```python
from build123d import *

# Parameters (mm, degrees)
SKETCH_1_R          = 4.75
EXTRUDE_1_DEPTH     = 7
CUT_EXTRUDE_1_DEPTH = 4
SKETCH_3_R          = 1.85
CUT_EXTRUDE_2_DEPTH = 8
CUT_EXTRUDE_7_DEPTH = 2.5


with BuildPart() as part:
    # Эскиз1 → Бобышка-Вытянуть1 (new body)
    with BuildSketch(Plane(origin=(0, 0, 0), x_dir=(1, 0, 0), z_dir=(0, 1, 0))):
        Circle(SKETCH_1_R)
    extrude(amount=EXTRUDE_1_DEPTH)

    # Эскиз2 → Вырез-Вытянуть1 (cut)
    with BuildSketch(Plane(origin=(0, 7, 0), x_dir=(1, 0, 0), z_dir=(0, 1, 0))):
        Polygon((-3.181980515, 0), (-2.25, -0.931980515), (-2.25, -2.25), (-0.931980515, -2.25), (0, -3.181980515), (0.931980515, -2.25), (2.25, -2.25), (2.25, -0.931980515), (3.181980515, 0), (2.25, 0.931980515), (2.25, 2.25), (0.931980515, 2.25), (0, 3.181980515), (-0.931980515, 2.25), (-2.25, 2.25), (-2.25, 0.931980515), align=None)
    extrude(amount=-CUT_EXTRUDE_1_DEPTH, mode=Mode.SUBTRACT)

    # Эскиз3 → Вырез-Вытянуть2 (cut, through all)
    with BuildSketch(Plane.XZ):
        Circle(SKETCH_3_R)
    extrude(amount=-CUT_EXTRUDE_2_DEPTH, mode=Mode.SUBTRACT)

    # Эскиз4<3> → Вырез-Вытянуть7 (cut)
    with BuildSketch(Plane.XZ):
        with BuildLine():
            ThreePointArc((2.254348542, 4.180958341), (-1.817746304, 4.388427779), (-4.550449136, 1.362318854))
            Line((-4.550449136, 1.362318854), (2.254348542, 4.180958341))
        make_face()
        with BuildLine():
            Line((4.550449136, -1.362318854), (-2.254348542, -4.180958341))
            ThreePointArc((-2.254348542, -4.180958341), (1.817746304, -4.388427779), (4.550449136, -1.362318854))
        make_face()
    extrude(amount=-CUT_EXTRUDE_7_DEPTH, mode=Mode.SUBTRACT)


solid = part.part
```
Verification items for the finished model (mm, model axes). A direction names the side the tool comes from. Round coordinates to 2 decimals unless told otherwise and drop trailing zeros. Order: outer loops, then holes, each group sorted by start corner. A loop starts at its lowest first (then second) coordinate and runs counter-clockwise, first axis right, second up. Notation, with made-up numbers: (21, 67.25) - (25, 67.25) arc R20 ccw to (25, 90.25) - close; hole circle Ø5 at (54.5, 23.25). An arc over 180 degrees is marked (long way). Use CSV: the item, a comma, the result in double quotes. Start each with the question number.
1) Section check C-C, the plane z = 1.5. Record the cut outline in (x, y), plus the area to 3 significant figures.
2) Section check D-D, the plane x = 2.5. Record the cut outline in (y, z), plus the area to 3 significant figures.
3) Section check B-B, the plane x = 1.5. Record the cut outline in (y, z), plus the area to 3 significant figures.
4) Section check A-A, the plane y = 5.5. Record the cut outline in (x, z), plus the area to 3 significant figures.
5) Go/stop test with flat-tipped pins: P1, Ø3, axis at y = 5, z = 2, coming from the +X side; P2, Ø2, axis at y = 4, z = -2.5, coming from the +X side; P3, Ø1, axis at x = -2, z = 3.5, coming from the -Y side; P4, Ø4.5, axis at x = 0, z = 0, coming from the -Y side. Record where each tip stops, or that it passes through.
6) Mould release check, pull along Z, two halves, no side actions. Record for faces 6 (the flat face through (1.2, 1.23, -2.75)), 7 (the flat face through (-1.2, 1.23, 2.75)), 8 (the flat face through (-2.2, 0, -0.1)), 9 (the flat face through (2.25, 5, 2)): +Z half, -Z half, draft (parallel to the pull), parting line (faces both ways), or undercut.
7) Thickness scan on L1, parallel to Z at x = 0, y = 0.85; L2, parallel to Y at x = 2.5, z = -0.5; L3, parallel to X at y = 3.5, z = -0.5. Record the ranges inside material, lowest first.
8) Access from +Z, -Z, +X, -X, +Y, -Y to the whole of each face (thin tool, end or side, straight path). Record for faces 1 (the cylindrical face through (-4.745, 4.229, -0.209)), 2 (the flat face through (3, 7, 1)), 3 (the flat face through (-1, 2.5, 3)), 4 (the flat face through (2, 5, 2.25)), 5 (the flat face through (1, 2.5, -3)).
Answers:
1,outline,"(-4.51, 2.5) - (-4.22, 2.5) - (-4.22, 0) - (-1.08, 0) - (-1.08, 3) - (-2.25, 3) - (-2.25, 7) - (-4.51, 7) - close; (1.08, 0) - (4.51, 0) - (4.51, 7) - (2.25, 7) - (2.25, 3) - (1.08, 3) - close"
1,area,"37.9 mm²"
2,outline,"(0, -2.21) - (2.5, -2.21) - (2.5, -4.04) - (7, -4.04) - (7, -0.68) - (3, -0.68) - (3, 0.68) - (7, 0.68) - (7, 4.04) - (0, 4.04) - close"
2,area,"46.5 mm²"
3,outline,"(0, -2.63) - (2.5, -2.63) - (2.5, -4.51) - (7, -4.51) - (7, -2.25) - (3, -2.25) - (3, -1.08) - (0, -1.08) - close; (0, 1.08) - (3, 1.08) - (3, 2.25) - (7, 2.25) - (7, 4.51) - (2.5, 4.51) - (2.5, 3.87) - (0, 3.87) - close"
3,area,"32.3 mm²"
4,outline,"circle Ø9.5 at (0, 0); hole (-3.18, 0) - (-2.25, -0.93) - (-2.25, -2.25) - (-0.93, -2.25) - (0, -3.18) - (0.93, -2.25) - (2.25, -2.25) - (2.25, -0.93) - (3.18, 0) - (2.25, 0.93) - (2.25, 2.25) - (0.93, 2.25) - (0, 3.18) - (-0.93, 2.25) - (-2.25, 2.25) - (-2.25, 0.93) - close"
4,area,"47.2 mm²"
5,P1,"stops at x = 4.72"
5,P2,"stops at x = 4.51"
5,P3,"stops at y = 2.5"
5,P4,"stops at y = 0"
6,face 6,"-Z half"
6,face 7,"+Z half"
6,face 8,"draft"
6,face 9,"undercut"
7,L1,"z = -3.25 to -1.85, 1.85 to 3.25"
7,L2,"y = 0 to 3"
7,L3,"x = -4.72 to -2.68, 2.68 to 4.72"
8,face 1,"+Y, -Y"
8,face 2,"+Z, -Z, +X, -X, +Y"
8,face 3,"+Z, -X, -Y"
8,face 4,"+Y"
8,face 5,"-Z, +X, -Y"
